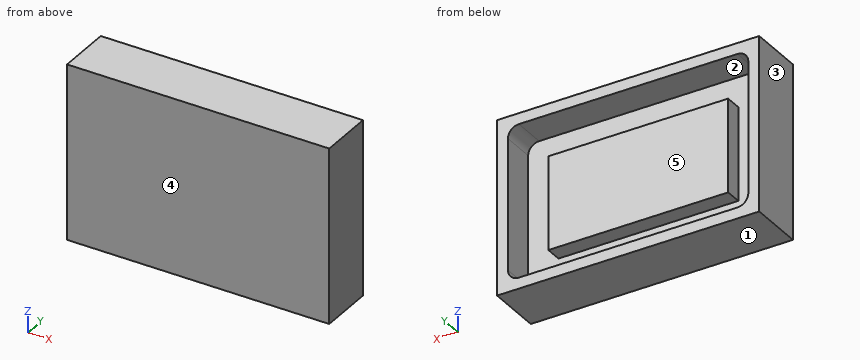
```python
from build123d import *

# Parameters (mm, degrees)
SKETCH4_W      = 76.2
SKETCH4_H      = 50.8
EXTRUDE2_DEPTH = 15.875
EXTRUDE3_DEPTH = 9.525
SKETCH6_W      = 52.256418226
SKETCH6_H      = 27.153557036
EXTRUDE4_DEPTH = 4.7625


with BuildPart() as part:
    # Sketch4 → Extrude2 (new body)
    with BuildSketch(Plane(origin=(0, 0, 0), x_dir=(1, 0, 0), z_dir=(0, 1, 0))):
        with Locations((38.1, 25.4)):
            Rectangle(SKETCH4_W, SKETCH4_H)
    extrude(amount=-EXTRUDE2_DEPTH)

    # Sketch5 → Extrude3 (cut)
    with BuildSketch(Plane(origin=(0, 0, 0), x_dir=(1, 0, 0), z_dir=(0, 1, 0))):
        with BuildLine():
            Line((3.175, 44.45), (3.175, 6.35))
            ThreePointArc((3.175, 6.35), (4.10493597, 4.10493597), (6.35, 3.175))
            Line((6.35, 3.175), (69.85, 3.175))
            ThreePointArc((69.85, 3.175), (72.09506403, 4.10493597), (73.025, 6.35))
            Line((73.025, 6.35), (73.025, 44.45))
            ThreePointArc((73.025, 44.45), (72.09506403, 46.69506403), (69.85, 47.625))
            Line((69.85, 47.625), (6.35, 47.625))
            ThreePointArc((6.35, 47.625), (4.10493597, 46.69506403), (3.175, 44.45))
        make_face()
    extrude(amount=-EXTRUDE3_DEPTH, mode=Mode.SUBTRACT)

    # Sketch6 → Extrude4 (add)
    with BuildSketch(Plane(origin=(0, -9.525, 0), x_dir=(-1, 0, 0), z_dir=(0, 1, 0))):
        with Locations((-38.1, -25.4)):
            Rectangle(SKETCH6_W, SKETCH6_H)
    extrude(amount=EXTRUDE4_DEPTH)


solid = part.part
```
Source: CAD feature listing. Evaluate the final solid. Frame: model axes, mm. Face numbers are marked on the shaded views. A direction names the side the tool comes from. Coordinates: 2 decimals unless noted, no trailing zeros. Loops run counter-clockwise (first coordinate to the right, second up) from the corner with the lowest first, then second, coordinate; pieces in that order, holes last. Notation, with made-up numbers: M -20.5,18.5 L 27.5,18.5 A16 ccw 27.5,23.5 Z; hole C 79,9.25 d11. An arc over 180 degrees is marked long. Use a Markdown table: item, result. Add a question column.
Q1. Section query A-A, the plane x = 49.5. Return loops of the section in (y, z) (1 decimal).
Q2. Draft query along Z for the marked faces 1, 2 and 3. Return one class per face: pulls with the +Z half, pulls with the -Z half, needs draft (parallel to the pull), parting line crosses it, or undercut.
Q3. First-contact query: pin 1 (8 mm diameter, centred on x = 32, z = -25.5, fed in from +Y). Flat tip, straight axial feed; report the tip coordinate or a pass-through.
Q4. Material intervals for L1, parallel to X at y = -7, z = -35.5 (3 decimals); L2, parallel to X at y = -0.5, z = -17 (3 decimals); L3, parallel to Z at x = 20.5, y = -2 (3 decimals), sorted ascending.
Q5. Section query C-C, the plane y = -2.75. Return loops of the section in (x, z) (3 decimals).
Q6. Section query B-B, the plane z = -40.5. Return loops of the section in (x, y) (3 decimals), and give its area (3 significant figures).
Q7. Section query D-D, the plane x = 68. Return loops of the section in (y, z) (3 decimals), and give its area (3 significant figures).
Q8. Access query for the marked faces 4 and 5. Directions: +Z, -Z, +X, -X, +Y, -Y. A direction counts if a zero-diameter tool reaches every point of the face in a straight line with its end or side. Return the directions, or none.
Result:
| question | item | result |
|---|---|---|
| 1 | outline | M -15.9,-50.8 L 0,-50.8 L 0,-47.6 L -9.5,-47.6 L -9.5,-39 L -4.8,-39 L -4.8,-11.8 L -9.5,-11.8 L -9.5,-3.2 L 0,-3.2 L 0,0 L -15.9,0 Z |
| 2 | face 1 | pulls with the -Z half |
| 2 | face 2 | undercut |
| 2 | face 3 | needs draft |
| 3 | pin 1 | stops at y = -4.76 |
| 4 | L1 | x = 0 to 3.175, 11.972 to 64.228, 73.025 to 76.2 |
| 4 | L2 | x = 0 to 3.175, 73.025 to 76.2 |
| 4 | L3 | z = -50.8 to -47.625, -3.175 to 0 |
| 5 | outline | M 0,-50.8 L 76.2,-50.8 L 76.2,0 L 0,0 Z; hole M 3.175,-44.45 A3.175 ccw 6.35,-47.625 L 69.85,-47.625 A3.175 ccw 73.025,-44.45 L 73.025,-6.35 A3.175 ccw 69.85,-3.175 L 6.35,-3.175 A3.175 ccw 3.175,-6.35 Z |
| 6 | outline | M 0,-15.875 L 76.2,-15.875 L 76.2,0 L 73.025,0 L 73.025,-9.525 L 3.175,-9.525 L 3.175,0 L 0,0 Z |
| 6 | area | 544 mm2 |
| 7 | outline | M -15.875,-50.8 L 0,-50.8 L 0,-47.625 L -9.525,-47.625 L -9.525,-3.175 L 0,-3.175 L 0,0 L -15.875,0 Z |
| 7 | area | 383 mm2 |
| 8 | face 4 | +Z, -Z, +X, -X, -Y |
| 8 | face 5 | +Y |
